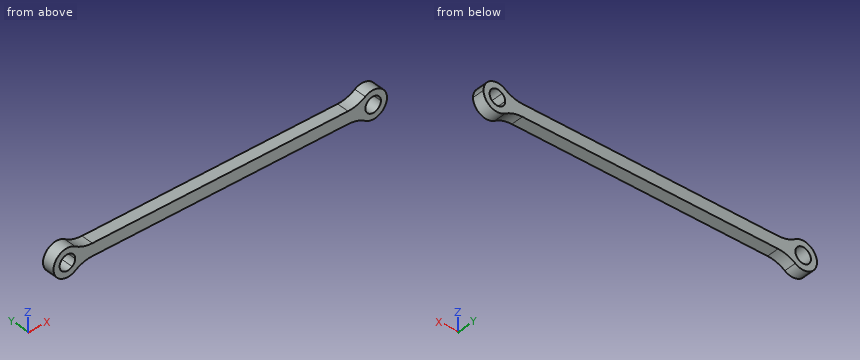
from build123d import *

# Parameters (mm, degrees)
BOSS_EXTRUDE1_DEPTH = 4
FILLET1_R           = 10


with BuildPart() as part:
    # Sketch1 → Boss-Extrude1 (new body)
    with BuildSketch(Plane(origin=(0, 0, 0), x_dir=(1, 0, 0), z_dir=(0, 1, 0))):
        with BuildLine():
            Line((-98.818070798, 2), (-96.313130783, 2))
            ThreePointArc((-96.313130783, 2), (-104.95, 0), (-96.313130783, -2))
            Line((-96.313130783, -2), (-98.818070798, -2))
            ThreePointArc((-98.818070798, -2), (-102.95, 0), (-98.818070798, 2))
        make_face()
        with BuildLine():
            Line((-4.55, 0), (-95.85, 0))
            ThreePointArc((-95.85, 0), (-95.967294565, -1.026461169), (-96.313130783, -2))
            Line((-96.313130783, -2), (-4.086869217, -2))
            ThreePointArc((-4.086869217, -2), (-4.432705435, -1.026461169), (-4.55, 0))
        make_face()
        with BuildLine():
            ThreePointArc((-96.313130783, 2), (-95.967294565, 1.026461169), (-95.85, 0))
            Line((-95.85, 0), (-4.55, 0))
            ThreePointArc((-4.55, 0), (-4.432705435, 1.026461169), (-4.086869217, 2))
            Line((-4.086869217, 2), (-96.313130783, 2))
        make_face()
        with BuildLine():
            Line((-97.85, 0), (-95.85, 0))
            ThreePointArc((-95.85, 0), (-95.967294565, 1.026461169), (-96.313130783, 2))
            Line((-96.313130783, 2), (-98.818070798, 2))
            ThreePointArc((-98.818070798, 2), (-98.104741903, 1.110986169), (-97.85, 0))
        make_face()
        with BuildLine():
            ThreePointArc((-96.313130783, -2), (-95.967294565, -1.026461169), (-95.85, 0))
            Line((-95.85, 0), (-97.85, 0))
            ThreePointArc((-97.85, 0), (-98.104741903, -1.110986169), (-98.818070798, -2))
            Line((-98.818070798, -2), (-96.313130783, -2))
        make_face()
        with BuildLine():
            ThreePointArc((4.55, 0), (1.026461169, 4.432705435), (-4.086869217, 2))
            Line((-4.086869217, 2), (-1.581929202, 2))
            ThreePointArc((-1.581929202, 2), (1.110986169, 2.295258097), (2.55, 0))
            ThreePointArc((2.55, 0), (1.110986169, -2.295258097), (-1.581929202, -2))
            Line((-1.581929202, -2), (-4.086869217, -2))
            ThreePointArc((-4.086869217, -2), (1.026461169, -4.432705435), (4.55, 0))
        make_face()
        with BuildLine():
            ThreePointArc((-4.086869217, 2), (-4.432705435, 1.026461169), (-4.55, 0))
            Line((-4.55, 0), (-2.55, 0))
            ThreePointArc((-2.55, 0), (-2.295258097, 1.110986169), (-1.581929202, 2))
            Line((-1.581929202, 2), (-4.086869217, 2))
        make_face()
        with BuildLine():
            Line((-2.55, 0), (-4.55, 0))
            ThreePointArc((-4.55, 0), (-4.432705435, -1.026461169), (-4.086869217, -2))
            Line((-4.086869217, -2), (-1.581929202, -2))
            ThreePointArc((-1.581929202, -2), (-2.295258097, -1.110986169), (-2.55, 0))
        make_face()
    extrude(amount=BOSS_EXTRUDE1_DEPTH)

    # Fillet1
    fillet1_edges = [part.edges().sort_by_distance(p)[0] for p in [
        (-4.086869217, 2, 2),
        (-96.313130783, 2, 2),
        (-96.313130783, 2, -2),
        (-4.086869217, 2, -2),
    ]]
    fillet(fillet1_edges, radius=FILLET1_R)


solid = part.part
Source: CAD feature listing. Evaluate the final solid. Frame: model axes, mm. Give positions to 0.01 mm unless a question says otherwise; leave off trailing zeros. Order: outer loops, then holes, each group sorted by start corner. A loop starts at its lowest first (then second) coordinate and runs counter-clockwise, first axis right, second up. Notation, with made-up numbers: (63.5, 25.25) -> (74.5, 25.25) arc R21 ccw to (74.5, 64.25) -> close; hole circle Ø2 at (13.25, -30.5). An arc over 180 degrees is marked (long way). Write item = value, one per line.
Item 1: Contact query for flat-ended pins moving along their axis: pin 1 (2 mm diameter, centred on x = -25, y = 2.5, fed in from +Z); pin 2 (1.5 mm diameter, centred on y = 3, z = -1.5, fed in from +X); pin 3 (2 mm diameter, centred on y = 2.5, z = -3, fed in from -X). Output: stop coordinate, or through.
Check result:
pin_1 = 2
pin_2 = 4.49
pin_3 = -104.49
Item 2: Section query A-A (y = 2.7). Output: boundary loops of the cut face in (x, z), then the cut area to 3 significant figures.
Check result:
outline = (-97.83, -3.75) arc R10 cw to (-92.17, -2) -> (-8.23, -2) arc R10 cw to (-2.57, -3.75) arc R4.55 ccw (long way) to (-2.57, 3.75) arc R10 cw to (-8.23, 2) -> (-92.17, 2) arc R10 cw to (-97.83, 3.75) arc R4.55 ccw (long way) to start; hole circle Ø5.1 at (-100.4, 0); hole circle Ø5.1 at (0, 0)
area = 462 mm²
Item 3: Ray query, probe 1 along Z at (x, y) = (-100.4, 1.75); probe 2 along X at (y, z) = (1.35, -0.25); probe 3 along X at (y, z) = (0.9, -1.25). Return the intervals inside material, ascending.
Check result:
probe_1 = -4.55 to -2.55, 2.55 to 4.55
probe_2 = -104.94 to -102.94, -97.86 to -2.54, 2.54 to 4.54
probe_3 = -104.77 to -102.62, -98.18 to -2.22, 2.22 to 4.37
Item 4: Section query B-B (x = -100.4). Output: boundary loops of the cut face in (y, z), then the cut area to 3 significant figures.
Check result:
outline = (0, -4.55) -> (4, -4.55) -> (4, -2.55) -> (0, -2.55) -> close; (0, 2.55) -> (4, 2.55) -> (4, 4.55) -> (0, 4.55) -> close
area = 16.0 mm²
Item 5: Section query D-D (x = -53.5). Output: boundary loops of the cut face in (y, z), then the cut area to 3 significant figures.
Check result:
outline = (0, -2) -> (4, -2) -> (4, 2) -> (0, 2) -> close
area = 16.0 mm²
Item 6: Section query C-C (z = 1). Output: boundary loops of the cut face in (x, y).
Check result:
outline = (-104.84, 0) -> (-102.75, 0) -> (-102.75, 4) -> (-104.84, 4) -> close; (-98.05, 0) -> (-2.35, 0) -> (-2.35, 4) -> (-98.05, 4) -> close; (2.35, 0) -> (4.44, 0) -> (4.44, 4) -> (2.35, 4) -> close
